```python
from build123d import *

# Parameters (mm, degrees)
BOSS_EXTRUDE1_DEPTH = 2.5
SKETCH2_R           = 1.5
CUT_EXTRUDE1_DEPTH  = 2.5


with BuildPart() as part:
    # Sketch1 → Boss-Extrude1 (new body)
    with BuildSketch(Plane.XY):
        with BuildLine():
            Line((7.6, -2.8), (7.6, -5.375))
            Line((7.6, -5.375), (-7.6, -5.375))
            Line((-7.6, -5.375), (-7.6, -2.8))
            Line((-7.6, -2.8), (-9.7, -2.8))
            ThreePointArc((-9.7, -2.8), (-12.5, 0), (-9.7, 2.8))
            Line((-9.7, 2.8), (-7.6, 2.8))
            Line((-7.6, 2.8), (-7.6, 5.375))
            Line((-7.6, 5.375), (7.6, 5.375))
            Line((7.6, 5.375), (7.6, 2.8))
            Line((7.6, 2.8), (9.7, 2.8))
            ThreePointArc((9.7, 2.8), (12.5, 0), (9.7, -2.8))
            Line((9.7, -2.8), (7.6, -2.8))
        make_face()
    extrude(amount=BOSS_EXTRUDE1_DEPTH)

    # Sketch2 → Cut-Extrude1 (cut)
    with BuildSketch(Plane.XY.offset(2.5)):
        with Locations((-9.7, 0)):
            Circle(SKETCH2_R)
        with Locations((9.7, 0)):
            Circle(SKETCH2_R)
    extrude(amount=-CUT_EXTRUDE1_DEPTH, mode=Mode.SUBTRACT)


solid = part.part
```
Geometry check sheet. Reference: the model listing, model coordinates, mm. A direction names the side the tool comes from. Round coordinates to 2 decimals unless told otherwise and drop trailing zeros. Write each loop counter-clockwise with the first axis right and the second up, starting at its lowest first coordinate (ties: lowest second). Pieces come first, ordered by that corner, then holes. Notation, with made-up numbers: (10, -5.5) - (43, -5.5) arc R28 cw to (43, 16.5) - close; hole circle Ø1 at (82.25, 69.25). An arc over 180 degrees is marked (long way). Write each question's results on one line, items separated by ' | '.
(1) Thickness scan on probe 1 along X at (y, z) = (-0.75, 2); probe 2 along Y at (x, z) = (-9.7, 1.15); probe 3 along X at (y, z) = (4.25, 1.4). Record the ranges inside material, lowest first. Write a range as from..to.
Computed:
probe 1: x = -12.4..-11, -8.4..8.4, 11..12.4 | probe 2: y = -2.8..-1.5, 1.5..2.8 | probe 3: x = -7.6..7.6
(2) Draft check along X on faces 6 (the face through (-7.6, 4, 1)), 7 (the face through (0, 5.375, 1)), 8 (the face through (-8.314, -0.575, 1.268)). Enter one of: pulls with the +X half, pulls with the -X half, needs draft (parallel to the pull), parting line crosses it, or undercut.
Computed:
face 6: pulls with the -X half | face 7: needs draft | face 8: undercut
(3) Sectioned sample at A-A, the plane y = 0. Enter the section's corners in (x, z).
Computed:
outline: (-12.5, 0) - (-11.2, 0) - (-11.2, 2.5) - (-12.5, 2.5) - close; (-8.2, 0) - (8.2, 0) - (8.2, 2.5) - (-8.2, 2.5) - close; (11.2, 0) - (12.5, 0) - (12.5, 2.5) - (11.2, 2.5) - close
(4) Set-up check for faces 1 (the face through (9, -2.8, 1)), 2 (the face through (-9, 2.8, 1)), 3 (the face through (9, 2.8, 1)), 4 (the face through (-9, -2.8, 1)), 5 (the face through (0, 0, 2.5)): record each of +Z, -Z, +X, -X, +Y, -Y from which the full face is reachable in a straight line by a thin tool's end or side.
Computed:
face 1: +Z, -Z, +X, -Y | face 2: +Z, -Z, -X, +Y | face 3: +Z, -Z, +X, +Y | face 4: +Z, -Z, -X, -Y | face 5: +Z, +X, -X, +Y, -Y
(5) Sectioned sample at C-C, the plane y = -4.5. Enter the section's corners in (x, z).
Computed:
outline: (-7.6, 0) - (7.6, 0) - (7.6, 2.5) - (-7.6, 2.5) - close
(6) Depth check by flat-ended pin: pin 1 Ø0.8 at (y, z) = (-4, 2) entering from +X; pin 2 Ø0.6 at (x, z) = (-9, 1.5) entering from +Y; pin 3 Ø1.8 at (x, y) = (-9.7, 0) entering from +Z; pin 4 Ø1.2 at (y, z) = (-3.5, 1.5) entering from -X. Enter the tip coordinate at first touch or a pass-through.
Computed:
pin 1: stops at x = 7.6 | pin 2: stops at y = 2.8 | pin 3: passes through | pin 4: stops at x = -7.6
(7) Sectioned sample at B-B, the plane z = 1.2. Enter the section's corners in (x, y) (3 decimals), plus the area to 3 significant figures.
Computed:
outline: (-9.7, -2.8) - (-7.6, -2.8) - (-7.6, -5.375) - (7.6, -5.375) - (7.6, -2.8) - (9.7, -2.8) arc R2.8 ccw to (9.7, 2.8) - (7.6, 2.8) - (7.6, 5.375) - (-7.6, 5.375) - (-7.6, 2.8) - (-9.7, 2.8) arc R2.8 ccw to start; hole circle Ø3 at (-9.7, 0); hole circle Ø3 at (9.7, 0) | area: 197 mm^2
